from build123d import *

# Parameters (mm, degrees)
SKETCH1_R           = 2
BOSS_EXTRUDE1_DEPTH = 1.5
SKETCH2_R           = 1.6
CUT_EXTRUDE1_DEPTH  = 1.5


with BuildPart() as part:
    # Sketch1 → Boss-Extrude1 (new body)
    with BuildSketch(Plane.XY):
        Polygon((-241.5, -120), (1.5, -120), (1.5, 10), (-161.5, 10), (-161.5, 1.5), (-241.5, 1.5), align=None)
        with Locations((-180.669950037, -60.870517352)):
            Circle(SKETCH1_R, mode=Mode.SUBTRACT)
    extrude(amount=BOSS_EXTRUDE1_DEPTH)

    # Sketch2 → Cut-Extrude1 (cut)
    with BuildSketch(Plane.XY.offset(1.5)):
        with Locations((-235, -5)):
            Circle(SKETCH2_R)
        with Locations((-235, -115)):
            Circle(SKETCH2_R)
        with Locations((-5, -115)):
            Circle(SKETCH2_R)
        with Locations((-120, 5)):
            Circle(SKETCH2_R)
        with Locations((-18.5, 5)):
            Circle(SKETCH2_R)
    extrude(amount=-CUT_EXTRUDE1_DEPTH, mode=Mode.SUBTRACT)


solid = part.part
Input: part model. Units: mm. Frame: model coordinates. Coordinates: 2 decimals unless noted, no trailing zeros. Loops run counter-clockwise (first coordinate to the right, second up) from the corner with the lowest first, then second, coordinate; pieces in that order, holes last. Notation, with made-up numbers: (-25.5, -27) - (-21.5, -27) arc R22 cw to (-21.5, -12) - close; hole circle Ø5 at (28.5, 79.25). An arc over 180 degrees is marked (long way). Answer in a Markdown table with one row per item. Add a question column.
Item 1: Line query: line 1 along Y through (x, z) = (-235, 1.1); line 2 along X through (y, z) = (-115, 1.05); line 3 along Y through (x, z) = (-5, 1.05). Output: solid intervals per line, ascending. Write a range as [from, to].
Item 2: Section query A-A on z = 0.35. Return the cut outline in (x, y).
Item 3: Section query B-B on x = -223. Return the cut outline in (y, z), then the cut area to 3 significant figures.
Item 4: Contact query for a flat-ended pin moving along its axis: P1, Ø4, axis at x = -51, y = -10.5, coming from the -Z side. Output: stop coordinate, or through.
Recorded:
| question | item | result |
|---|---|---|
| 1 | line 1 | [-120, -116.6], [-113.4, -6.6], [-3.4, 1.5] |
| 1 | line 2 | [-241.5, -236.6], [-233.4, -6.6], [-3.4, 1.5] |
| 1 | line 3 | [-120, -116.6], [-113.4, 10] |
| 2 | outline | (-241.5, -120) - (1.5, -120) - (1.5, 10) - (-161.5, 10) - (-161.5, 1.5) - (-241.5, 1.5) - close; hole circle Ø3.2 at (-235, -115); hole circle Ø3.2 at (-235, -5); hole circle Ø4 at (-180.67, -60.87); hole circle Ø3.2 at (-120, 5); hole circle Ø3.2 at (-18.5, 5); hole circle Ø3.2 at (-5, -115) |
| 3 | outline | (-120, 0) - (1.5, 0) - (1.5, 1.5) - (-120, 1.5) - close |
| 3 | area | 182 mm^2 |
| 4 | P1 | z = 0 |
